Model file for the job. Use its own axes, mm. A direction names the side the tool comes from. Coordinates: 2 decimals unless noted, no trailing zeros. Loops run counter-clockwise (first coordinate to the right, second up) from the corner with the lowest first, then second, coordinate; pieces in that order, holes last. Notation, with made-up numbers: (-23.75, -31) -> (-2.75, -31) arc R21 cw to (-2.75, 4) -> close; hole circle Ø1 at (43.5, 79.25). An arc over 180 degrees is marked (long way). Use one line per item in the form item = value.
Autodesk Inventor part; units mm, degrees
ref_plane "YZ Plane" through (0, 0, 0) normal (1, 0, 0) x (0, 1, 0)
ref_plane "XZ Plane" through (0, 0, 0) normal (0, 1, 0) x (-1, 0, 0)
ref_plane "XY Plane" through (0, 0, 0) normal (0, 0, 1) x (1, 0, 0)
sketch "スケッチ1" plane through (0, 0, 0) normal (0, 0, 1) x (1, 0, 0)
  line L0 (0, 0) -> (18, 0)
  line L1 (18, 0) -> (18, 18)
  line L2 (18, 18) -> (0, 18)
  line L3 (0, 18) -> (0, 0)
  line L4 (0, 13.7574) -> (4.2426, 18)
  line L5 (0, 13.7574) -> (6, 13.7574) construction
  line L6 (4.2426, 0) -> (0, 4.2426)
  line L7 (18, 4.2426) -> (13.7574, 0)
  line L8 (13.7574, 18) -> (18, 13.7574)
  point P0 (0, 9)
  point P1 (9, 18)
  point P2 (9, 9)
  dimension "d0" = 18
  dimension "d1" = 18
  dimension "d2" = 45
  dimension "d3" = 3
  dimension "d13" = 9
  dimension "d14" = 9
  dimension "d17" = 360
extrude "押し出し1" add sketch "スケッチ1" along normal blind 9.5 contours L6 L3 L4 L2 L8 L1 L7 L0
sketch "スケッチ2" plane through (0, 0, 9.5) normal (0, 0, 1) x (1, 0, 0)
  line L0 (0, 0) -> (13.7574, 0)
  line L1 (0, 13.7574) -> (0, 0)
  circle A0 centre (9, 9) radius 8.7
  point P0 (9, 0)
  point P1 (5.6569, 0)
  point P2 (12.3431, 0)
  point P3 (0, 9.7071)
  point P4 (0, 5.6569)
  point P5 (18, 0)
  point P6 (0, 18)
  dimension "d10" = 17.4
extrude "押し出し2" add sketch "スケッチ2" along normal blind 55
sketch "スケッチ3" plane through (9, 9, 64.5) normal (0, 0, 1) x (1, 0, 0)
  circle A0 centre (0, 0) radius 8.7
  line L0 (4.7574, 9) -> (-4.7574, 9)
  line L1 (-4.7574, 9) -> (-9, 4.7574)
  line L2 (-9, 4.7574) -> (-9, -4.7574)
  line L3 (-9, -4.7574) -> (-4.7574, -9)
  line L4 (-4.7574, -9) -> (4.7574, -9)
  line L5 (4.7574, -9) -> (9, -4.7574)
  line L6 (9, -4.7574) -> (9, 4.7574)
  line L7 (9, 4.7574) -> (4.7574, 9)
  point P0 (-9, -9)
extrude "押し出し3" add sketch "スケッチ3" along normal blind 12.5 contours A0 | L7 L6 L5 L4 L3 L2 L1 L0
sketch "スケッチ4" plane through (9, 9, 77) normal (0, 0, 1) x (1, 0, 0)
  circle A0 centre (0, 0) radius 8.7
  circle A1 centre (0, 0) radius 5
  point P0 (-9, -9)
  dimension "d21" = 10
extrude "押し出し4" add sketch "スケッチ4" along normal blind 8 contours A1
sketch "スケッチ5" plane through (9, 9, 85) normal (0, 0, 1) x (1, 0, 0)
  circle A0 centre (0, 0) radius 5
  circle A1 centre (0, 0) radius 3
  point P0 (-9, -9)
  dimension "d24" = 6
extrude "押し出し5" cut sketch "スケッチ5" against normal blind 70 contours A1
properties part number "airclinder_30" material "アルミニウム 6061-AHC"
Q1. Which spindle directions (+Z, -Z, +X, -X, +Y, -Y) get a long thin tool onto all of the face, cutting with end or side? Do faces 5 (the face through (13, 5, 77)), 6 (the face through (2.59, 3.12, 36.61)), 7 (the face through (2.09, 2.15, 70.66)). Say none if no direction does.
Result:
face_5 = +Z
face_6 = none
face_7 = +Z, -Z, -X, -Y
Q2. Band-saw the part on C-C, the plane z = 7. Write the cut outline in (x, y).
Result:
outline = (0, 4.24) -> (4.24, 0) -> (13.76, 0) -> (18, 4.24) -> (18, 13.76) -> (13.76, 18) -> (4.24, 18) -> (0, 13.76) -> close
Q3. Band-saw the part on B-B, the plane z = 74. Write the cut outline in (x, y), and give its area (3 significant figures).
Result:
outline = (0, 4.24) -> (4.24, 0) -> (13.76, 0) -> (18, 4.24) -> (18, 13.76) -> (13.76, 18) -> (4.24, 18) -> (0, 13.76) -> close; hole circle Ø6 at (9, 9)
area = 260 mm2
Q4. Wall check: line 1 along Y through (x, z) = (9, 51.5); line 2 along Z through (x, y) = (15, 2.75); line 3 along Z through (x, y) = (9.5, 7.75). Give the ranges that are in metal, low to high.
Result:
line_1 = 0.3 to 6, 12 to 17.7
line_2 = 0 to 77
line_3 = 0 to 15
Q5. Mould opens along Y. For faces 1 (the face through (15.85, 2.09, 70.66)), 2 (the face through (9, 9, 15)), 3 (the face through (11.77, 7.85, 50.49)), 4 (the face through (0, 9, 5)) say: released by +Y, released by -Y, zero draft, split by the parting line, or undercut.
Result:
face_1 = released by -Y
face_2 = undercut
face_3 = undercut
face_4 = zero draft
Q6. Pin check, flat tips, straight feed: pin 1 Ø2 at (x, z) = (7, 14) entering from +Y; pin 2 Ø8 at (y, z) = (16, 18.5) entering from -X; pin 3 Ø4 at (x, z) = (11, 29.5) entering from +Y. Stop position of each tip, or through.
Result:
pin_1 = 17.64
pin_2 = 0.83
pin_3 = 17.7
Q7. Band-saw the part on A-A, the plane y = 9. Write the cut outline in (x, z), and give its area (3 significant figures).
Result:
outline = (0, 0) -> (18, 0) -> (18, 9.5) -> (17.7, 9.5) -> (17.7, 64.5) -> (18, 64.5) -> (18, 77) -> (14, 77) -> (14, 85) -> (12, 85) -> (12, 15) -> (6, 15) -> (6, 85) -> (4, 85) -> (4, 77) -> (0, 77) -> (0, 64.5) -> (0.3, 64.5) -> (0.3, 9.5) -> (0, 9.5) -> close
area = 1,010 mm2
